from build123d import *

# Parameters (mm, degrees)
SKETCH_1_R      = 1.6
SKETCH_1_W      = 5
SKETCH_1_H      = 3
EXTRUDE_3_DEPTH = 3


with BuildPart() as part:
    # 草图1 → 凸台-拉伸3 (new body)
    with BuildSketch(Plane(origin=(0, 0, 0), x_dir=(1, 0, 0), z_dir=(0, 1, 0))):
        with BuildLine():
            Line((-64.620407451, -23), (-64.620407451, 0))
            Line((-64.620407451, 0), (-61.620407451, 0))
            Line((-61.620407451, 0), (-61.620407451, -6))
            Line((-61.620407451, -6), (-58.620407451, -6))
            Line((-58.620407451, -6), (-58.620407451, 7.279592288))
            Line((-58.620407451, 7.279592288), (-52.620407451, 7.279592288))
            Line((-52.620407451, 7.279592288), (-52.620407451, 4.279592288))
            Line((-52.620407451, 4.279592288), (-55.620407451, 4.279592288))
            Line((-55.620407451, 4.279592288), (-55.620407451, 0))
            Line((-55.620407451, 0), (-22.120407451, 0))
            Line((-22.120407451, 0), (-22.120407451, -6))
            Line((-22.120407451, -6), (-19.120407451, -6))
            Line((-19.120407451, -6), (-19.120407451, 0))
            Line((-19.120407451, 0), (8.058394468, 0))
            Line((8.058394468, 0), (8.058394468, 3.112438553))
            Line((8.058394468, 3.112438553), (10.879592549, 3.112438553))
            Line((10.879592549, 3.112438553), (10.879592549, -6))
            Line((10.879592549, -6), (13.879592549, -6))
            Line((13.879592549, -6), (13.879592549, 0))
            Line((13.879592549, 0), (28.379592549, 0))
            Line((28.379592549, 0), (28.379592549, 3.112438553))
            Line((28.379592549, 3.112438553), (25.370412077, 3.112438553))
            Line((25.370412077, 3.112438553), (25.370412077, 6.112438553))
            Line((25.370412077, 6.112438553), (28.379592549, 6.112438553))
            Line((28.379592549, 6.112438553), (28.379592549, 12.612438553))
            Line((28.379592549, 12.612438553), (38.379592549, 12.612438553))
            Line((38.379592549, 12.612438553), (38.379592549, -13))
            ThreePointArc((38.379592549, -13), (35.450660361, -20.071067812), (28.379592549, -23))
            Line((28.379592549, -23), (13.879592549, -23))
            Line((13.879592549, -23), (13.879592549, -16))
            Line((13.879592549, -16), (10.879592549, -16))
            Line((10.879592549, -16), (10.879592549, -23))
            Line((10.879592549, -23), (-19.120407451, -23))
            Line((-19.120407451, -23), (-19.120407451, -16))
            Line((-19.120407451, -16), (-22.120407451, -16))
            Line((-22.120407451, -16), (-22.120407451, -23))
            Line((-22.120407451, -23), (-58.620407451, -23))
            Line((-58.620407451, -23), (-58.620407451, -16))
            Line((-58.620407451, -16), (-61.620407451, -16))
            Line((-61.620407451, -16), (-61.620407451, -23))
            Line((-61.620407451, -23), (-64.620407451, -23))
        make_face()
        with Locations(Location((-60.120407451, -11, 0), (0, 0, 270))):
            Circle(SKETCH_1_R, mode=Mode.SUBTRACT)
        with Locations(Location((-20.620407451, -11, 0), (0, 0, 270))):
            Circle(SKETCH_1_R, mode=Mode.SUBTRACT)
        with Locations(Location((12.379592549, -11, 0), (0, 0, 270))):
            Circle(SKETCH_1_R, mode=Mode.SUBTRACT)
        with Locations((33.379592549, 9.548629934)):
            Rectangle(SKETCH_1_W, SKETCH_1_H, mode=Mode.SUBTRACT)
    extrude(amount=-EXTRUDE_3_DEPTH)


solid = part.part
Geometry check sheet. Reference: the model listing, model coordinates, mm. A direction names the side the tool comes from. Give positions to 0.01 mm unless a question says otherwise; leave off trailing zeros. Order: outer loops, then holes, each group sorted by start corner. A loop starts at its lowest first (then second) coordinate and runs counter-clockwise, first axis right, second up.
1) Material ranges on probe 1 along X at (y, z) = (-2.3, 10.5); probe 2 along X at (y, z) = (-0.75, 11); probe 3 along X at (y, z) = (-2.5, -2), recorded low to high.
Results are:
probe 1: x = -64.62 to -61.64, -58.6 to -22.14, -19.1 to 10.86, 13.9 to 38.38
probe 2: x = -64.62 to -61.72, -58.52 to -22.22, -19.02 to 10.78, 13.98 to 38.38
probe 3: x = -58.62 to -55.62, 8.06 to 10.88, 28.38 to 38.38
2) Cross-section at A-A (z = 2). Record the boundary of the cut face in (x, y), then the cut area to 3 significant figures.
Results are:
outline: (-64.62, -3) - (-61.62, -3) - (-61.62, 0) - (-64.62, 0) - close; (-58.62, -3) - (-22.12, -3) - (-22.12, 0) - (-58.62, 0) - close; (-19.12, -3) - (10.88, -3) - (10.88, 0) - (-19.12, 0) - close; (13.88, -3) - (38.38, -3) - (38.38, 0) - (13.88, 0) - close
area: 282 mm2
3) Gauge pin test, flat ends, axial feed: pin 1 (0.9 mm diameter, centred on x = -32.5, y = -1.5, fed in from -Z); pin 2 (1.5 mm diameter, centred on y = -1, z = -1, fed in from -X); pin 3 (0.9 mm diameter, centred on x = -57, y = -1, fed in from -Z). Record the tip position at first contact, or that the pin passes through.
Results are:
pin 1: stops at z = 0
pin 2: stops at x = -58.62
pin 3: stops at z = -7.28
4) Cross-section at C-C (z = 11). Record the boundary of the cut face in (x, y), then the cut area to 3 significant figures.
Results are:
outline: (-64.62, -3) - (-61.72, -3) - (-61.72, 0) - (-64.62, 0) - close; (-58.52, -3) - (-22.22, -3) - (-22.22, 0) - (-58.52, 0) - close; (-19.02, -3) - (10.78, -3) - (10.78, 0) - (-19.02, 0) - close; (13.98, -3) - (38.38, -3) - (38.38, 0) - (13.98, 0) - close
area: 280 mm2
5) Draft check along X on faces 6 (the flat face through (33, -1, -11.049)), 7 (the flat face through (38.38, -1, 0)), 8 (the flat face through (-4, -1, 23)). Enter one of: released by +X, released by -X, zero draft, split by the parting line, or undercut.
Results are:
face 6: undercut
face 7: released by +X
face 8: zero draft
6) Cross-section at D-D (y = -1.3). Give the number of separate pieces and of enclosed holes in the cut face, then the cut area to 3 significant figures.
Results are:
separate pieces: 1
enclosed holes: 4
area: 2,370 mm2
7) Cross-section at B-B (x = -5.5). Record the boundary of the cut face in (y, z), then the cut area to 3 significant figures.
Results are:
outline: (-3, 0) - (0, 0) - (0, 23) - (-3, 23) - close
area: 69.0 mm2
8) Tool access check on faces 1 (the flat face through (35.88, -1, -10)), 2 (the flat face through (-12, 0, 9)), 3 (the flat face through (-63, -1, 23)), 4 (the flat face through (-61.62, -1, 19)), 5 (the flat face through (25.37, -1, -5)). Record the directions out of +Z, -Z, +X, -X, +Y, -Y that give a thin tool (end or side, any length) a straight path to the whole face; none if there is none.
Results are:
face 1: +Y, -Y
face 2: +Z, -Z, +X, -X, +Y
face 3: +Z, +X, -X, +Y, -Y
face 4: +Z, +Y, -Y
face 5: -Z, +Y, -Y
